Can you work these out from the model? Positions are in its coordinate system, mm. Coordinates: 2 decimals unless noted, no trailing zeros. Loops run counter-clockwise (first coordinate to the right, second up) from the corner with the lowest first, then second, coordinate; pieces in that order, holes last.
```python
from build123d import *

# Parameters (mm, degrees)
BOSS_EXTRUDE1_DEPTH = 4
SKETCH2_R           = 20
SKETCH2_R_2         = 12.5
SKETCH2_R_3         = 15
SKETCH2_R_4         = 7.5
BOSS_EXTRUDE2_DEPTH = 7.5


with BuildPart() as part:
    # Sketch1 → Boss-Extrude1 (new, symmetric)
    with BuildSketch(Plane.XY):
        with BuildLine():
            Line((59.81488788, 13.727342811), (-199.220649297, 19.976731751))
            ThreePointArc((-199.220649297, 19.976731751), (-185.706002057, 13.796933419), (-180.18511212, 0))
            ThreePointArc((-180.18511212, 0), (-185.84170962, -13.937962718), (-199.611792592, -19.991780929))
            Line((-199.611792592, -19.991780929), (59.81488788, -16.272657189))
            ThreePointArc((59.81488788, -16.272657189), (44.81488788, -1.272657189), (59.81488788, 13.727342811))
        make_face()
    extrude(amount=BOSS_EXTRUDE1_DEPTH, both=True)

    # Sketch2 → Boss-Extrude2 (add, symmetric)
    # profile 1 of 2: a face of its own
    with BuildSketch(Plane.XY):
        with Locations((-200.18511212, 0)):
            Circle(SKETCH2_R)
        with Locations((-200.18511212, 0)):
            Circle(SKETCH2_R_2, mode=Mode.SUBTRACT)
    # profile 2 of 2: a face of its own
    with BuildSketch(Plane.XY):
        with Locations((59.81488788, -1.272657189)):
            Circle(SKETCH2_R_3)
        with Locations((59.81488788, -1.272657189)):
            Circle(SKETCH2_R_4, mode=Mode.SUBTRACT)
    extrude(amount=BOSS_EXTRUDE2_DEPTH, both=True)


solid = part.part
```
Item 1: I need wall thicknesses on line 1 along X through (y, z) = (-2, -3.25); line 2 along X through (y, z) = (2, 2); line 3 along Z through (x, y) = (-4, 4). Which ranges of each line are inside material? Lowest first, please.
Results are:
line 1: x = -220.08 to -212.52, -187.85 to 52.35, 67.28 to 74.8
line 2: x = -220.08 to -212.52, -187.85 to 53.07, 66.56 to 74.45
line 3: z = -4 to 4
Item 2: I'm going to push flat-ended pins straight in: P1, Ø6, axis at x = 5.5, z = 1.5, coming from the -Y side; P2, Ø8, axis at x = -173, z = -5.5, coming from the +Y side; P3, Ø4, axis at y = 7.5, z = -0.5, coming from the -X side. Where does each tip first touch, or does it pass through?
Results are:
P1: stops at y = -17.09
P2: stops at y = 19.43
P3: stops at x = -219.41
Item 3: Suppose I cut it at B-B, the plane x = -73. Please give me the cut outline in (y, z).
Results are:
outline: (-18.18, -4) - (16.93, -4) - (16.93, 4) - (-18.18, 4) - close
Item 4: We'd pull the mould along X, two halves only. Please class faces 1 (the face through (-200, -13, -7.5)), 2 (the face through (66.97, 0.98, -0.11)), 3 (the face through (74.122, 3.233, 0.105)): +X half, -X half, draft (parallel to the pull), parting line (faces both ways), or undercut.
Results are:
face 1: draft
face 2: undercut
face 3: undercut
Item 5: Suppose I cut it at A-A, the plane x = -39. Please give me the cut outline in (y, z).
Results are:
outline: (-17.69, -4) - (16.11, -4) - (16.11, 4) - (-17.69, 4) - close
